For this review, take the finished solid that the model builds, in its own axes (mm). A direction names the side the tool comes from. Coordinates: 2 decimals unless noted, no trailing zeros. Loops run counter-clockwise (first coordinate to the right, second up) from the corner with the lowest first, then second, coordinate; pieces in that order, holes last. Notation, with made-up numbers: (73.5, 37) - (95.5, 37) arc R16 ccw to (95.5, 57) - close; hole circle Ø5 at (48.5, 7.5). An arc over 180 degrees is marked (long way). Use one line per item in the form item = value. Start each with the question number.
1. Add section D-D on z = 3.5. Give the boundary of the cut face in (x, y).
2. Add section B-B on y = 1.75. Give the boundary of the cut face in (x, z).
3. Draft analysis for pull direction Z (two halves, no side actions). For faces 1 (the face through (-18.95, 1.48, 8.09)), 2 (the face through (7, 10, 1)), 3 (the face through (-1, 1, -8.849)), state which applies: +Z half, -Z half, draft (parallel to the pull), parting line (faces both ways), or undercut.
4. To check wall thickness, follow probe 1 along Y at (x, z) = (15, -6.75); probe 2 along X at (y, z) = (4, 7); probe 3 along X at (y, z) = (9.75, 2). State the ranges of each line that lie inside material, in increasing order.
5. Add section C-C on x = 8.5. Give the boundary of the cut face in (y, z), and give its area (3 significant figures).
6. Machinability: for faces 4 (the face through (-1, 0, 1)), 5 (the face through (5.923, 6.451, 8.473)), which of the approach directions +Z, -Z, +X, -X, +Y, -Y give a long, thin tool a straight path to every point of the face, cutting with its end or side? Answer none if there is none.
7. Add section A-A on z = 7.75. Give the boundary of the cut face in (x, y).
8. For pin 1 Ø2 at (x, z) = (-16, -1) entering from +Y; pin 2 Ø2 at (x, y) = (-5, 4.5) entering from -Z; pin 3 Ø3.5 at (x, z) = (16.55, -5.85) entering from +Y; pin 4 Ø3 at (x, y) = (-8, 6) entering from +Z, all flat-tipped, find the tip position at first contact; note any pin that passes through.
```python
from build123d import *

# Parameters (mm, degrees)
SKETCH1_W           = 40
SKETCH1_H           = 20
SKETCH1_R           = 1.5
SKETCH1_R_2         = 7.5
BOSS_EXTRUDE1_DEPTH = 3
SKETCH1_2_R         = 7.5
BOSS_EXTRUDE2_DEPTH = 10


with BuildPart() as part:
    # Sketch1 → Boss-Extrude1 (new body)
    with BuildSketch(Plane(origin=(0, 0, 0), x_dir=(1, 0, 0), z_dir=(0, 1, 0))):
        with Locations((-0.451467269, -1.151241535)):
            Rectangle(SKETCH1_W, SKETCH1_H)
        with Locations((-17.451467269, 5.848758465)):
            Circle(SKETCH1_R, mode=Mode.SUBTRACT)
        with Locations((-17.451467269, -8.151241535)):
            Circle(SKETCH1_R, mode=Mode.SUBTRACT)
        with Locations((-8.451467269, -1.151241535)):
            Circle(SKETCH1_R_2, mode=Mode.SUBTRACT)
        with Locations((16.548532731, -8.151241535)):
            Circle(SKETCH1_R, mode=Mode.SUBTRACT)
        with Locations((16.548532731, 5.848758465)):
            Circle(SKETCH1_R, mode=Mode.SUBTRACT)
        with Locations((7.548532731, -1.151241535)):
            Circle(SKETCH1_R_2, mode=Mode.SUBTRACT)
    extrude(amount=BOSS_EXTRUDE1_DEPTH)

    # Sketch1<2> → Boss-Extrude2 (add)
    with BuildSketch(Plane(origin=(0, 0, 0), x_dir=(1, 0, 0), z_dir=(0, 1, 0))):
        with Locations((-8.451467269, -1.151241535)):
            Circle(SKETCH1_2_R)
        with Locations((7.548532731, -1.151241535)):
            Circle(SKETCH1_2_R)
    extrude(amount=BOSS_EXTRUDE2_DEPTH)


solid = part.part
```
Conclusion:
q1.outline = (-20.45, 0) - (19.55, 0) - (19.55, 3) - (14.67, 3) - (14.67, 10) - (0.43, 10) - (0.43, 3) - (-1.33, 3) - (-1.33, 10) - (-15.57, 10) - (-15.57, 3) - (-20.45, 3) - close
q2.outline = (-20.45, -8.85) - (19.55, -8.85) - (19.55, 11.15) - (-20.45, 11.15) - close; hole circle Ø3 at (-17.45, -5.85); hole circle Ø3 at (-17.45, 8.15); hole circle Ø3 at (16.55, -5.85); hole circle Ø3 at (16.55, 8.15)
q3.face_1 = undercut
q3.face_2 = draft
q3.face_3 = -Z half
q4.probe_1 = 0 to 3
q4.probe_2 = -13.15 to -3.76, 2.85 to 12.24
q4.probe_3 = -15.9 to -1, 0.1 to 15
q5.outline = (0, -8.85) - (3, -8.85) - (3, -6.29) - (10, -6.29) - (10, 8.59) - (3, 8.59) - (3, 11.15) - (0, 11.15) - close
q5.area = 164 mm^2
q6.face_4 = +Z, -Z, +X, -X, -Y
q6.face_5 = +Y
q7.outline = (-20.45, 0) - (-18.9, 0) - (-18.9, 3) - (-20.45, 3) - close; (-16.01, 0) - (15.1, 0) - (15.1, 3) - (11.11, 3) - (11.11, 10) - (3.98, 10) - (3.98, 3) - (-4.89, 3) - (-4.89, 10) - (-12.02, 10) - (-12.02, 3) - (-16.01, 3) - close; (17.99, 0) - (19.55, 0) - (19.55, 3) - (17.99, 3) - close
q8.pin_1 = 10
q8.pin_2 = -5.94
q8.pin_3 = 3
q8.pin_4 = 8.65
